Read the model definition and answer for the solid it produces. Units are mm, in the model's axes. Face numbers are marked on the shaded views. A direction names the side the tool comes from. Coordinates: 2 decimals unless noted, no trailing zeros. Loops run counter-clockwise (first coordinate to the right, second up) from the corner with the lowest first, then second, coordinate; pieces in that order, holes last. Notation, with made-up numbers: M -3.75,-27.5 L 33.25,-27.5 A31 ccw 33.25,11.5 Z; hole C -4,-34 d6. An arc over 180 degrees is marked long. One line per item, written item: value. Start each with the question number.
1. Flat-ended cylindrical pins translate along their axes: pin 1 (1 mm diameter, centred on x = -5, z = -64, fed in from -Y); pin 2 (2.5 mm diameter, centred on x = -5, z = -63, fed in from +Y); pin 3 (3.5 mm diameter, centred on x = 5, z = -64, fed in from +Y). Find the tip coordinate at first contact, or state that the pin passes through.
2. The part is cut by section A-A (z = -64). Write down the section's boundary in (x, y) (3 decimals), then the cut area to 3 significant figures.
3. For the marked faces 1, 2 and 3, determine the directions among +Z, -Z, +X, -X, +Y, -Y from which every point of the face is accessible in a straight line to the end or side of a thin tool.
4. Consider probe 1 along Y at (x, z) = (0, -59) (3 decimals); probe 2 along Z at (x, y) = (-7.5, -3.75); probe 3 along Y at (x, z) = (-2.75, -56). Determine where each line is inside the solid, lowest interval first.
5. The part is cut by section B-B (z = -39). Write down the section's boundary in (x, y) (1 decimal).
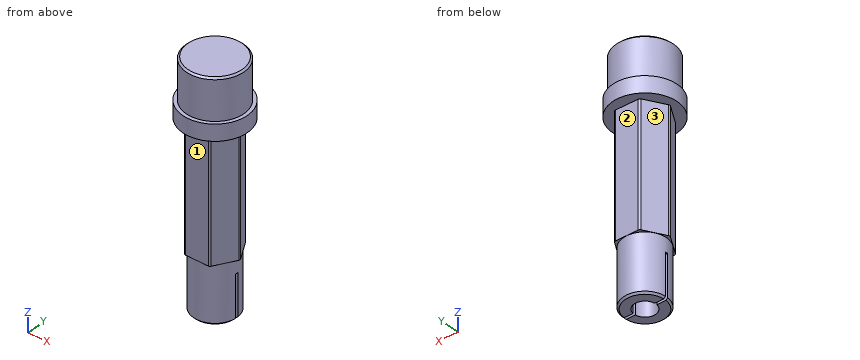
```python
from build123d import *

# Parameters (mm, degrees)
SKETCH2_OUTSIDE_W  = 35.99
SKETCH2_OUTSIDE_H  = 35.99
CUT_EXTRUDE1_DEPTH = 36.07435
FILLET1_R          = 0.635
CUT_EXTRUDE2_START = -12.7
CUT_EXTRUDE2_DEPTH = 12.7
CHAMFER1_SIZE      = 0.508


with BuildPart() as part:
    # Sketch1 → Revolve1 (revolve)
    with BuildSketch(Plane(origin=(0, 0, 0), x_dir=(0, 0, -1), z_dir=(1, 0, 0)), mode=Mode.PRIVATE) as revolve1_sk:
        Polygon((0, 0), (0, 8.5), (12, 8.5), (12, 9.525), (16.7625, 9.525), (16.7625, 7.62), (40.08605, 7.62), (52.83685, 7.62), (52.83685, 6.35), (69.67705, 6.35), (69.67705, 3.175), (54.43705, 3.175), (52.529317535, 0), align=None)
    revolve(revolve1_sk.sketch.rotate(Axis((0, 0, 0), (0, 0, 1)), 90), axis=Axis((0, 0, 0), (0, 0, 1)))

    # Sketch2 outside → Cut-Extrude1 (cut)
    with BuildSketch(Plane(origin=(0, 0, -16.7625), x_dir=(-1, 0, 0), z_dir=(0, 0, -1))):
        Rectangle(SKETCH2_OUTSIDE_W, SKETCH2_OUTSIDE_H)
        Polygon((3.696970073, 6.40334), (-3.696970073, 6.40334), (-7.393940145, 0), (-3.696970073, -6.40334), (3.696970073, -6.40334), (7.393940145, 0), align=None, mode=Mode.SUBTRACT)
    extrude(amount=CUT_EXTRUDE1_DEPTH, mode=Mode.SUBTRACT)

    # Fillet1
    fillet1_edges = [part.edges().sort_by_distance(p)[0] for p in [
        (-7.393940145, 0, -34.799675),
        (-3.696970073, -6.40334, -34.799675),
        (3.696970073, -6.40334, -34.799675),
        (7.393940145, 0, -34.799675),
        (3.696970073, 6.40334, -34.799675),
        (-3.696970073, 6.40334, -34.799675),
    ]]
    fillet(fillet1_edges, radius=FILLET1_R)

    # Sketch3 → Cut-Extrude2 (cut)
    with BuildSketch(Plane(origin=(0, 0, -69.67705), x_dir=(-1, 0, 0), z_dir=(0, 0, -1)).offset(CUT_EXTRUDE2_START)):
        with BuildLine():
            Line((-8.998734144, 0.381), (-3.152057106, 0.381))
            ThreePointArc((-3.152057106, 0.381), (0, 3.175), (3.152057106, 0.381))
            Line((3.152057106, 0.381), (8.998734144, 0.381))
            Line((8.998734144, 0.381), (8.998734144, -0.381))
            Line((8.998734144, -0.381), (3.152057106, -0.381))
            ThreePointArc((3.152057106, -0.381), (0, -3.175), (-3.152057106, -0.381))
            Line((-3.152057106, -0.381), (-8.998734144, -0.381))
            Line((-8.998734144, -0.381), (-8.998734144, 0.381))
        make_face()
    extrude(amount=CUT_EXTRUDE2_DEPTH, mode=Mode.SUBTRACT)

    # Chamfer1
    chamfer1_edges = [part.edges().sort_by_distance(p)[0] for p in [
        (0, 6.35, -69.67705),
        (8.5, 0, 0),
        (0, -6.35, -69.67705),
    ]]
    chamfer(chamfer1_edges, length=CHAMFER1_SIZE)


solid = part.part
```
Answer block:
1. pin 1: stops at y = -4.48
1. pin 2: stops at y = 5.12
1. pin 3: stops at y = 5.46
2. outline: M -6.339,-0.381 A6.35 ccw 6.339,-0.381 L 3.152,-0.381 A3.175 cw -3.152,-0.381 Z; M -6.339,0.381 L -3.152,0.381 A3.175 cw 3.152,0.381 L 6.339,0.381 A6.35 ccw Z
2. area: 90.2 mm2
3. face 1: -Z, +X, -X, -Y
3. face 2: -Z, +X, -X, +Y
3. face 3: -Z, -X, +Y
4. probe 1: y = -6.35 to -3.175, 3.175 to 6.35
4. probe 2: z = -16.76 to -0.39
4. probe 3: y = -5.72 to -1.59, 1.59 to 5.72
5. outline: M -7.2,-0.3 L -3.9,-6.1 A0.6 ccw -3.3,-6.4 L 3.3,-6.4 A0.6 ccw 3.9,-6.1 L 7.2,-0.3 A0.6 ccw 7.2,0.3 L 3.9,6.1 A0.6 ccw 3.3,6.4 L -3.3,6.4 A0.6 ccw -3.9,6.1 L -7.2,0.3 A0.6 ccw Z
